Design review of the part built by this model. Coordinates are the model's own, in mm. A direction names the side the tool comes from. Coordinates: 2 decimals unless noted, no trailing zeros. Loops run counter-clockwise (first coordinate to the right, second up) from the corner with the lowest first, then second, coordinate; pieces in that order, holes last. Notation, with made-up numbers: (44, 61) - (61, 61) arc R15 cw to (61, 66) - close; hole circle Ø1 at (4, 39.25). An arc over 180 degrees is marked (long way). Answer in a Markdown table with one row per item. Add a question column.
(1) We need section A-A, the plane y = 58.5. Write out the cut boundary in (x, z), plus the area to 3 significant figures.
(2) To check wall thickness, follow L1, parallel to Y at x = 5.5, z = 5; L2, parallel to Y at x = 17.1, z = 3.1; L3, parallel to X at y = 26, z = 7.5. State the ranges of each line that lie inside material, in increasing order. Write a range as [from, to].
(3) We need section D-D, the plane z = 4.75. Write out the cut boundary in (x, y).
(4) We need section B-B, the plane z = 1. Give the number of separate pieces and of enclosed holes in the cut face, plus the area to 3 significant figures.
(5) Clearance check with a flat-ended pin moving along its axis: pin 1 (6 mm diameter, centred on x = 45, y = 34.5, fed in from +Z). State where the tip first meets the part, or that it passes through.
(6) For faces 4 (the face through (56.9, 32, 6)), 5 (the face through (45.15, 36.87, 1.97)), list the 3-axis set-ups (+Z, -Z, +X, -X, +Y, -Y) from which the entire face can be reached by the end or side of a thin tool; tool diameter is ignored.
(7) The part is to be moulded in two halves that separate along Y. For faces 1 (the face through (0.57, 0.6, 4.06)), 2 (the face through (47.12, 46.948, 6.028)), 3 (the face through (32, 64, 4)), say which applies: released by +Y, released by -Y, zero draft, split by the parting line, or undercut.
Autodesk Inventor part; units mm, degrees
ref_plane "YZ Plane" through (0, 0, 0) normal (1, 0, 0) x (0, 1, 0)
ref_plane "XZ Plane" through (0, 0, 0) normal (0, 1, 0) x (-1, 0, 0)
ref_plane "XY Plane" through (0, 0, 0) normal (0, 0, 1) x (1, 0, 0)
sketch "スケッチ1" plane through (0, 0, 0) normal (0, 0, 1) x (1, 0, 0)
  line L0 (0, 0) -> (64, 0)
  line L1 (64, 0) -> (64, 64)
  line L2 (64, 64) -> (0, 64)
  line L3 (0, 64) -> (0, 0)
  line L4 (5.5, 58.5) -> (58.5, 58.5) construction
  line L5 (58.5, 58.5) -> (58.5, 5.5) construction
  line L6 (58.5, 5.5) -> (5.5, 5.5) construction
  line L7 (5.5, 5.5) -> (5.5, 58.5) construction
  circle A0 centre (5.5, 58.5) radius 1.75
  circle A1 centre (5.5, 5.5) radius 1.75
  circle A2 centre (58.5, 5.5) radius 1.75
  circle A3 centre (58.5, 58.5) radius 1.75
  line L8 (0, 32) -> (64, 32) construction
  line L9 (32, 64) -> (32, 0) construction
  line L10 (17.1, 27.05) -> (46.9, 27.05) construction
  line L11 (46.9, 27.05) -> (46.9, 36.95) construction
  line L12 (46.9, 36.95) -> (17.1, 36.95) construction
  line L13 (17.1, 36.95) -> (17.1, 27.05) construction
  line L14 (17.1, 27.05) -> (46.9, 36.95) construction
  line L15 (46.9, 27.05) -> (17.1, 36.95) construction
  circle A4 centre (46.9, 36.95) radius 1.75
  circle A5 centre (46.9, 27.05) radius 1.75
  circle A6 centre (17.1, 27.05) radius 1.75
  circle A7 centre (17.1, 36.95) radius 1.75
  point P0 (32, 32)
  dimension "d0" = 64
  dimension "d2" = 53
  dimension "d3" = 3.5
  dimension "d4" = 3.5
  dimension "d5" = 9.9
  dimension "d6" = 29.8
extrude "押し出し1" add sketch "スケッチ1" along normal blind 8
fillet "フィレット1" radius 2 4 edges at (0, 0, 4) (64, 0, 4) (64, 64, 4) (0, 64, 4)
sketch "スケッチ2" plane through (0, 0, 8) normal (0, 0, 1) x (1, 0, 0)
  circle A0 centre (17.1, 36.95) radius 1.75
  circle A1 centre (17.1, 27.05) radius 1.75
  line L0 (17.1, 36.95) -> (17.1, 27.05) construction
  line L1 (7.1, 36.95) -> (7.1, 27.05)
  line L2 (27.1, 27.05) -> (27.1, 36.95)
  arc A2 (27.1, 36.95) -> (7.1, 36.95) centre (17.1, 36.95) ccw
  arc A3 (7.1, 27.05) -> (27.1, 27.05) centre (17.1, 27.05) ccw
  circle A4 centre (46.9, 36.95) radius 1.75
  circle A5 centre (46.9, 27.05) radius 1.75
  line L3 (46.9, 36.95) -> (46.9, 27.05) construction
  line L4 (36.9, 36.95) -> (36.9, 27.05)
  line L5 (56.9, 27.05) -> (56.9, 36.95)
  arc A6 (56.9, 36.95) -> (36.9, 36.95) centre (46.9, 36.95) ccw
  arc A7 (36.9, 27.05) -> (56.9, 27.05) centre (46.9, 27.05) ccw
  point P0 (0, 0)
  point P1 (17.1, 32)
  point P2 (46.9, 32)
  dimension "d10" = 10
  dimension "d11" = 10
extrude "押し出し2" cut sketch "スケッチ2" against normal blind 4
properties part number "_3D プリント"
Responses:
| question | item | result |
|---|---|---|
| 1 | outline | (0, 0) - (3.75, 0) - (3.75, 8) - (0, 8) - close; (7.25, 0) - (56.75, 0) - (56.75, 8) - (7.25, 8) - close; (60.25, 0) - (64, 0) - (64, 8) - (60.25, 8) - close |
| 1 | area | 456 mm2 |
| 2 | L1 | y = [0, 3.75], [7.25, 56.75], [60.25, 64] |
| 2 | L2 | y = [0, 25.3], [28.8, 35.2], [38.7, 64] |
| 2 | L3 | x = [0, 7.16], [27.04, 36.96], [56.84, 64] |
| 3 | outline | (0, 2) arc R2 ccw to (2, 0) - (62, 0) arc R2 ccw to (64, 2) - (64, 62) arc R2 ccw to (62, 64) - (2, 64) arc R2 ccw to (0, 62) - close; hole circle Ø3.5 at (5.5, 5.5); hole circle Ø3.5 at (5.5, 58.5); hole (7.1, 27.05) arc R10 ccw to (27.1, 27.05) - (27.1, 36.95) arc R10 ccw to (7.1, 36.95) - close; hole (36.9, 27.05) arc R10 ccw to (56.9, 27.05) - (56.9, 36.95) arc R10 ccw to (36.9, 36.95) - close; hole circle Ø3.5 at (58.5, 5.5); hole circle Ø3.5 at (58.5, 58.5) |
| 4 | separate pieces | 1 |
| 4 | enclosed holes | 8 |
| 4 | area | 4,020 mm2 |
| 5 | pin 1 | stops at z = 4 |
| 6 | face 4 | +Z |
| 6 | face 5 | +Z, -Z |
| 7 | face 1 | released by -Y |
| 7 | face 2 | undercut |
| 7 | face 3 | released by +Y |
